from build123d import *

# Parameters (mm, degrees)
F1_DEPTH        = 12.7
F2_R            = 9.525
F3_SIZE         = 1.524
F4_R            = 1.016
F6_DEPTH        = 2
F7_R            = 6.35
F8_R            = 3.175
F10_DEPTH       = 3.001
F12_D           = 4.4958
F12_DEPTH       = 25.4
F12_CSINK_D     = 9.1186
F12_CSINK_ANGLE = 82
F12_TIP         = 1.3506745855


# Not quite as in the source:
# - a pattern or mirror of a feature is missing from the dataset's text; its kind, count and spacing are read off the source's solid


with BuildPart() as f1:
    # F0 (on Right) → F1 (new body, symmetric)
    with BuildSketch(Plane.YZ):
        Polygon((3, 40), (0, 40), (0, 0), (40, 0), (40, 3), (3, 3), align=None)
    extrude(amount=F1_DEPTH, both=True)

    # F2
    f2_edges = [f1.edges().sort_by_distance(p)[0] for p in [
        (0, 3, 3),
    ]]
    fillet(f2_edges, radius=F2_R)

    # F3
    f3_edges = [f1.edges().sort_by_distance(p)[0] for p in [
        (0, 0, 0),
    ]]
    chamfer(f3_edges, length=F3_SIZE)

    # F4
    f4_edges = [f1.edges().sort_by_distance(p)[0] for p in [
        (0, 0, 1.524),
        (0, 1.524, 0),
    ]]
    fillet(f4_edges, radius=F4_R)

    # F5 (on face) → F6 (join)
    with BuildSketch(Plane.YZ.offset(12.7)):
        with BuildLine():
            Line((33.65, 0), (0, 33.65))
            Line((0, 33.65), (0, 1.9448409794))
            ThreePointArc((0, 1.9448409794), (0.077338395, 1.5560346121), (0.2975795103, 1.2264204897))
            Line((0.2975795103, 1.2264204897), (1.2264204897, 0.2975795103))
            ThreePointArc((1.2264204897, 0.2975795103), (1.5560346121, 0.077338395), (1.9448409794, 0))
            Line((1.9448409794, 0), (33.65, 0))
        make_face()
    f6 = extrude(amount=-F6_DEPTH)

    # F6_copies: F6 across plane
    add(f6.mirror(Plane(origin=(0, 0, 0), x_dir=(0, 0, -1), z_dir=(-1, 0, 0))))

    # F7
    f7_edges = [f1.edges().sort_by_distance(p)[0] for p in [
        (12.7, 1.5, 40),
        (-12.7, 1.5, 40),
        (-12.7, 40, 1.5),
        (12.7, 40, 1.5),
    ]]
    fillet(f7_edges, radius=F7_R)

    # F8
    f8_edges = [f1.edges().sort_by_distance(p)[0] for p in [
        (11.7, 3, 30.65),
        (11.7, 30.65, 3),
        (-11.7, 30.65, 3),
        (-11.7, 3, 30.65),
    ]]
    fillet(f8_edges, radius=F8_R)

    # F9 (on face) → F10 (cut, through all)
    with BuildSketch(Plane(origin=(0, 3, 0), x_dir=(-1, 0, 0), z_dir=(0, 1, 0))):
        with BuildLine():
            Line((1.75, 22), (1.75, 30))
            ThreePointArc((1.75, 30), (0, 28.25), (-1.75, 30))
            Line((-1.75, 30), (-1.75, 22))
            ThreePointArc((-1.75, 22), (0, 23.75), (1.75, 22))
        make_face()
        with BuildLine():
            ThreePointArc((-1.75, 30), (0, 28.25), (1.75, 30))
            ThreePointArc((1.75, 30), (0, 31.75), (-1.75, 30))
        make_face()
        with BuildLine():
            ThreePointArc((-1.75, 22), (0, 20.25), (1.75, 22))
            ThreePointArc((1.75, 22), (0, 23.75), (-1.75, 22))
        make_face()
    extrude(amount=-F10_DEPTH, mode=Mode.SUBTRACT)

    # F12
    with Locations(Plane.XY.offset(3)):
        with Locations((0, 26.2625)):
            CounterSinkHole(F12_D / 2, F12_CSINK_D / 2, depth=F12_DEPTH, counter_sink_angle=F12_CSINK_ANGLE)
            with Locations((0, 0, -(F12_DEPTH + F12_TIP / 2))):  # 118° drill point
                Cone(0, F12_D / 2, F12_TIP, mode=Mode.SUBTRACT)


solid = f1.part
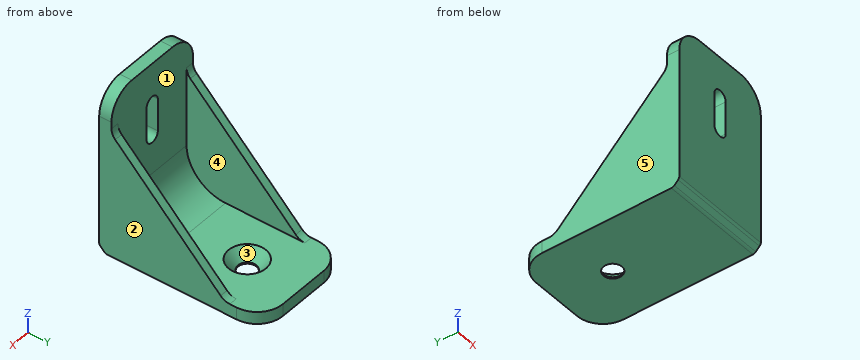
Work out the finished part from the listing and answer in its coordinate system (mm). Face numbers are marked on the shaded views. A direction names the side the tool comes from. Give positions to 0.01 mm unless a question says otherwise; leave off trailing zeros. Write each loop counter-clockwise with the first axis right and the second up, starting at its lowest first coordinate (ties: lowest second). Pieces come first, ordered by that corner, then holes. Notation, with made-up numbers: (76, -32) - (86, -32) arc R37 cw to (86, 6) - close; hole circle Ø7 at (26, 65). An arc over 180 degrees is marked (long way). One line per item, written item: value. Start each with the question number.
1. Find section B-B (x = 0). Write down the section's boundary in (y, z) (3 decimals).
2. For a pull along Y with two mould halves and no side action, classify the marked faces 1, 2 and 3 as +Y half, -Y half, draft (parallel to the pull), parting line (faces both ways), or undercut.
3. Find section D-D (y = 19). Write down the section's boundary in (x, z), then the cut area to 3 significant figures.
4. Given pin 1 (2 mm diameter, centred on x = 9, z = 11, fed in from +Y); pin 2 (3.5 mm diameter, centred on x = 0, y = 26.26, fed in from -Z); pin 3 (4 mm diameter, centred on x = 6.5, y = 12, fed in from +Z); pin 4 (12.5 mm diameter, centred on x = 2, z = 28, fed in from +Y), each flat-ended and moving along its own axis, determine where each tip first touches the part or whether it passes through.
5. Find section C-C (z = 18.5). Write down the section's boundary in (x, y), then the cut area to 3 significant figures.
6. For the marked faces 4 and 5, determine the directions among +Z, -Z, +X, -X, +Y, -Y from which every point of the face is accessible in a straight line to the end or side of a thin tool.
7. Find section A-A (z = 26). Write down the section's boundary in (x, y).
8. Consider probe 1 along X at (y, z) = (27.5, 3.5); probe 2 along Y at (x, z) = (-5.5, 35.5). Determine where each line is inside the solid, lowest interval first.
Geometry results:
1. outline: (0, 1.945) arc R1.016 ccw to (0.298, 1.226) - (1.226, 0.298) arc R1.016 ccw to (1.945, 0) - (24.015, 0) - (24.015, 0.341) - (21.703, 3) - (12.525, 3) arc R9.525 cw to (3, 12.525) - (3, 20.25) - (0, 20.25) - close; (0, 31.75) - (3, 31.75) - (3, 40) - (0, 40) - close; (28.51, 0) - (40, 0) - (40, 3) - (30.822, 3) - (28.51, 0.341) - close
2. face 1: +Y half
2. face 2: draft
2. face 3: undercut
3. outline: (-12.7, 0) - (12.7, 0) - (12.7, 14.65) - (10.7, 14.65) - (10.7, 3) - (-10.7, 3) - (-10.7, 14.65) - (-12.7, 14.65) - close
3. area: 123 mm2
4. pin 1: y = 3.34
4. pin 2: through
4. pin 3: z = 3.34
4. pin 4: y = 3
5. outline: (-12.7, 0) - (12.7, 0) - (12.7, 15.15) - (10.7, 15.15) - (10.7, 3) - (-10.7, 3) - (-10.7, 15.15) - (-12.7, 15.15) - close
5. area: 125 mm2
6. face 4: +Z, +Y
6. face 5: +Z, -Z, -X, +Y, -Y
7. outline: (-12.7, 0) - (-1.75, 0) - (-1.75, 3) - (-10.7, 3) - (-10.7, 7.65) - (-12.7, 7.65) - close; (1.75, 0) - (12.7, 0) - (12.7, 7.65) - (10.7, 7.65) - (10.7, 3) - (1.75, 3) - close
8. probe 1: -12.7 to -10.7, 10.7 to 12.7
8. probe 2: 0 to 3
